```python
from build123d import *

# Parameters (mm, degrees)
F1_DEPTH = 30
F2_W     = 11
F2_H     = 15
F3_DEPTH = 11
F4_W     = 15
F4_H     = 8
F5_DEPTH = 11
F6_ANGLE = -90
F8_DEPTH = 11.001


with BuildPart() as f1:
    # F0 (on Front) → F1 (new body)
    with BuildSketch(Plane.XZ):
        Polygon((0, 30), (0, 0), (40, 0), (40, 11), (11, 11), (11, 30), align=None)
    extrude(amount=F1_DEPTH)

    # F2 (on face) → F3 (cut, through all)
    with BuildSketch(Plane.XY.offset(11)):
        with Locations((34.5, -22.5)):
            Rectangle(F2_W, F2_H)
    extrude(amount=-F3_DEPTH, mode=Mode.SUBTRACT)

    # F4 (on face) → F5 (cut, through all)
    with BuildSketch(Plane.YZ.offset(11)):
        with Locations((-22.5, 26)):
            Rectangle(F4_W, F4_H)
    extrude(amount=-F5_DEPTH, mode=Mode.SUBTRACT)


with BuildPart() as f1_1:
    # F6: moved
    add(f1.part.rotate(Axis((0, 0, 15), (0, 0, 1)), F6_ANGLE))

    # F7 (on face) → F8 (cut, through all)
    with BuildSketch(Plane.XZ.offset(11)):
        Polygon((-7.5, 26), (-15, 30), (-15, 22), align=None)
        Polygon((0, 30), (-15, 30), (-7.5, 26), align=None)
    extrude(amount=-F8_DEPTH, mode=Mode.SUBTRACT)


solid = f1_1.part
```
CAD build for the part. Positions are in the model's coordinates, mm. A direction names the side the tool comes from. Round coordinates to 2 decimals unless told otherwise and drop trailing zeros. Loops run counter-clockwise (first coordinate to the right, second up) from the corner with the lowest first, then second, coordinate; pieces in that order, holes last. Notation, with made-up numbers: (12, 47) - (66, 47) arc R20 ccw to (66, 56) - close; hole circle Ø4 at (47, -40). An arc over 180 degrees is marked (long way). Return JSON: item names as keys, results as strings. Group by question number.
Q1. Flat gauge pins, fed straight in: pin 1 Ø5.5 at (x, z) = (-21.5, 24) entering from -Y; pin 2 Ø2 at (x, y) = (-11, -31) entering from +Z; pin 3 Ø5.5 at (x, z) = (-21.5, 3.5) entering from -Y. Where does each tip first touch, or does it go through?
Q2. Band-saw the part on C-C on z = 6.5. Give the cut face in (x, y), plus the area to 4 significant figures.
Q3. Band-saw the part on A-A on y = -9.5. Give the cut face in (x, z).
Q4. Drill centre lines: line 1 along Y through (x, z) = (-11, 19.75); line 2 along Z through (x, y) = (-10, -23); line 3 along Z through (x, y) = (-16, -6). Where is each one in solid material? Low to high. Write a range as [from, to].
Q5. Tool access for faces 1 (the face through (-23, -6, 22)), 2 (the face through (-15, -34, 6)), 3 (the face through (-15, -22, 11)), 4 (the face through (-15, 0, 12)): list every direction of +Z, -Z, +X, -X, +Y, -Y with a clear straight run to the whole face (end or side of a thin tool).
Q6. Band-saw the part on B-B on x = -6. Give the cut face in (y, z), plus the area to 3 significant figures.
Q7. Band-saw the part on D-D on z = 14. Give the cut face in (x, y), plus the area to 3 significant figures.
Solutions:
{
 "1": {"pin 1": "stops at y = -11", "pin 2": "stops at z = 11", "pin 3": "stops at y = -29"},
 "2": {"outline": "(-30, -29) - (-15, -29) - (-15, -40) - (0, -40) - (0, 0) - (-30, 0) - close", "area": "1,035 mm^2"},
 "3": {"outline": "(-30, 0) - (0, 0) - (0, 30) - (-15, 22) - (-30, 22) - close"},
 "4": {"line 1": "y = [-11, 0]", "line 2": "z = [0, 11]", "line 3": "z = [0, 22]"},
 "5": {"face 1": "+Z, -X, +Y, -Y", "face 2": "+Z, -Z, -X, -Y", "face 3": "+Z, +X, -X, -Y", "face 4": "+Z, -Z, +X, -X, +Y"},
 "6": {"outline": "(-40, 0) - (0, 0) - (0, 26.8) - (-11, 26.8) - (-11, 11) - (-40, 11) - close", "area": "614 mm^2"},
 "7": {"outline": "(-30, -11) - (0, -11) - (0, 0) - (-30, 0) - close", "area": "330 mm^2"}
}
